Build history of the part. All positions in model axes, mm. A direction names the side the tool comes from. Give positions to 0.01 mm unless a question says otherwise; leave off trailing zeros. Loops run counter-clockwise (first coordinate to the right, second up) from the corner with the lowest first, then second, coordinate; pieces in that order, holes last.
1) Wall check: line 1 (Y direction, x = -10, z = 3.9); line 2 (X direction, y = 7.5, z = 3); line 3 (Y direction, x = 3.5, z = 3.95). Give the ranges that are in metal, low to high.
2) Band-saw the part on A-A on z = 3. State how many separate pieces and enclosed holes the cut face has, then the cut area to 3 significant figures.
3) 3-axis set-ups, long thin cutter, end or side, ignore diameter. For faces 1 (the flat face through (9, 3.5, 3)), 2 (the flat face through (-9, -3.5, 3)), 3 (the flat face through (-9, 3.5, 3)): which of +Z, -Z, +X, -X, +Y, -Y reach the whole face in a straight line?
4) Band-saw the part on C-C on x = 2.5. List the corners of the cut face in (y, z).
5) Band-saw the part on D-D on z = 0.5. List the corners of the cut face in (x, y).
6) Two-plate mould, pull along Z, no slides. Class faces 4 (the cylindrical face through (0, -8, 3)), 5 (the cylindrical face through (3.254, 10.678, 3.169)), 6 (the flat face through (-4, 5, 0)): +Z half, -Z half, draft (parallel to the pull), parting line (faces both ways), or undercut.
7) Flat gauge pins, fed straight in: P1, Ø2, axis at x = -0.5, z = 3, coming from the +Y side; P2, Ø2, axis at x = -10, y = 0, coming from the +Z side; P3, Ø1.3, axis at x = 9.5, z = 2.5, coming from the -Y side; P4, Ø0.5, axis at x = -9.5, z = 3, coming from the +Y side. Where does each tip first touch, or does it go through?
8) Band-saw the part on B-B on y = 7.25. List the corners of the cut face in (x, z).
```python
from build123d import *

# Parameters (mm, degrees)
SKETCH1_R           = 1.3
BOSS_EXTRUDE1_DEPTH = 6
SKETCH2_R           = 1.3
CUT_EXTRUDE1_DEPTH  = 11


with BuildPart() as part:
    # Sketch1 → Boss-Extrude1 (new body)
    with BuildSketch(Plane.XY):
        with BuildLine():
            Line((-10, 3.5), (-8.351646544, 3.5))
            ThreePointArc((-8.351646544, 3.5), (-7.402963246, 3.739318314), (-6.681317235, 4.4))
            ThreePointArc((-6.681317235, 4.4), (-6.080676089, 5.198593877), (-5.385164807, 5.916079783))
            Line((-5.385164807, 5.916079783), (-5.444775123, 5.916079783))
            Line((-5.444775123, 5.916079783), (-5.444775123, 12.916079783))
            Line((-5.444775123, 12.916079783), (-1, 12.916079783))
            Line((-1, 12.916079783), (-1, 5.916079783))
            ThreePointArc((-1, 5.916079783), (0, -6), (1, 5.916079783))
            Line((1, 5.916079783), (1, 12.916079783))
            Line((1, 12.916079783), (5.444775123, 12.916079783))
            Line((5.444775123, 12.916079783), (5.444775123, 5.861264698))
            ThreePointArc((5.444775123, 5.861264698), (6.106910233, 5.16775071), (6.681317235, 4.4))
            ThreePointArc((6.681317235, 4.4), (7.402963246, 3.739318314), (8.351646544, 3.5))
            Line((8.351646544, 3.5), (10, 3.5))
            ThreePointArc((10, 3.5), (13.5, 0), (10, -3.5))
            Line((10, -3.5), (8.351646544, -3.5))
            ThreePointArc((8.351646544, -3.5), (7.402963246, -3.739318314), (6.681317235, -4.4))
            ThreePointArc((6.681317235, -4.4), (0, -8), (-6.681317235, -4.4))
            ThreePointArc((-6.681317235, -4.4), (-7.402963246, -3.739318314), (-8.351646544, -3.5))
            Line((-8.351646544, -3.5), (-10, -3.5))
            ThreePointArc((-10, -3.5), (-13.5, 0), (-10, 3.5))
        make_face()
        with Locations((-10, 0)):
            Circle(SKETCH1_R, mode=Mode.SUBTRACT)
        with Locations((10, 0)):
            Circle(SKETCH1_R, mode=Mode.SUBTRACT)
    extrude(amount=BOSS_EXTRUDE1_DEPTH)

    # Sketch2 → Cut-Extrude1 (cut)
    with BuildSketch(Plane(origin=(5.444775123, 0, 0), x_dir=(0, 0, -1), z_dir=(1, 0, 0))):
        with Locations((-3, 9.388672241)):
            Circle(SKETCH2_R)
    extrude(amount=-CUT_EXTRUDE1_DEPTH, mode=Mode.SUBTRACT)


solid = part.part
```
Findings below:
1. line 1: y = -3.5 to -1.3, 1.3 to 3.5
1. line 2: x = -5.44 to -1, 1 to 5.44
1. line 3: y = -7.19 to -4.87, 4.87 to 8.5, 10.28 to 12.92
2. separate pieces: 3
2. enclosed holes: 2
2. area: 172 mm2
3. face 1: +Z, -Z, +X, +Y
3. face 2: +Z, -Z, -X, -Y
3. face 3: +Z, -Z, -X, +Y
4. outline: (-7.6, 0) - (-5.45, 0) - (-5.45, 6) - (-7.6, 6) - close; (5.45, 0) - (12.92, 0) - (12.92, 6) - (5.45, 6) - close; hole circle Ø2.6 at (9.39, 3)
5. outline: (-10, -3.5) - (-8.35, -3.5) arc R2 cw to (-6.68, -4.4) arc R8 ccw to (6.68, -4.4) arc R2 cw to (8.35, -3.5) - (10, -3.5) arc R3.5 ccw to (10, 3.5) - (8.35, 3.5) arc R2 cw to (6.68, 4.4) arc R8 ccw to (5.44, 5.86) - (5.44, 12.92) - (1, 12.92) - (1, 5.92) arc R6 cw (long way) to (-1, 5.92) - (-1, 12.92) - (-5.44, 12.92) - (-5.44, 5.92) - (-5.39, 5.92) arc R8 ccw to (-6.68, 4.4) arc R2 cw to (-8.35, 3.5) - (-10, 3.5) arc R3.5 ccw to start; hole circle Ø2.6 at (-10, 0); hole circle Ø2.6 at (10, 0)
6. face 4: draft
6. face 5: undercut
6. face 6: -Z half
7. P1: stops at y = 12.92
7. P2: passes through
7. P3: stops at y = -3.5
7. P4: stops at y = 3.5
8. outline: (-5.44, 0) - (-1, 0) - (-1, 6) - (-5.44, 6) - close; (1, 0) - (5.44, 0) - (5.44, 6) - (1, 6) - close
